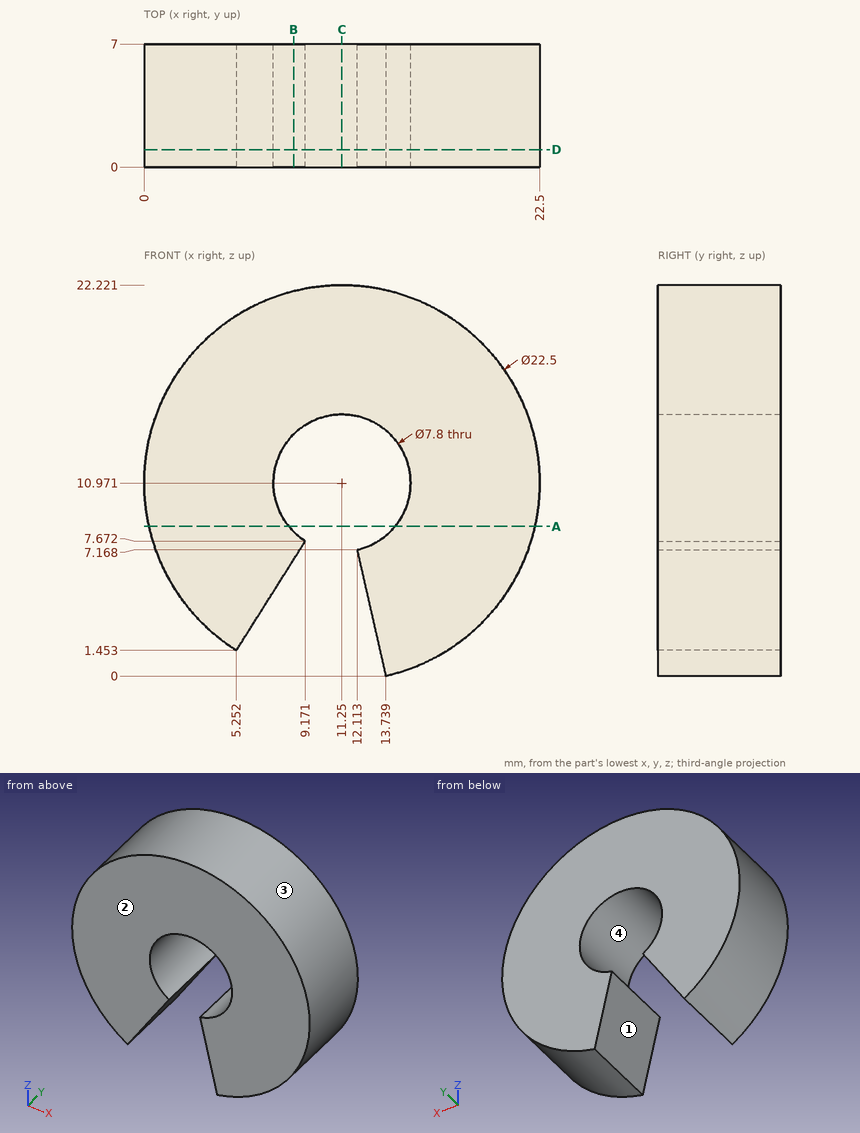
Geometry check sheet. Reference: drawing and pictorial views, mm from the part's lowest x, y, z. Coordinates: 2 decimals unless noted, no trailing zeros. Order: outer loops, then holes, each group sorted by start corner. A loop starts at its lowest first (then second) coordinate and runs counter-clockwise, first axis right, second up.
Item 1: Section check A-A (z = 8.5). Enter the section's corners in (x, y) (1 decimal).
Item 2: Mould release check, pull along Z, two halves, no side actions. Record for the marked faces 1, 2, 3 and 4: released by +Z, released by -Z, zero draft, split by the parting line, or undercut.
Item 3: Section check B-B (x = 8.5). Enter the section's corners in (y, z) (1 decimal).
Item 4: Scan lines: line 1 along Z through (x, y) = (11.25, 2.75); line 2 along Z through (x, y) = (8.75, 3.75) (1 decimal); line 3 along X through (y, z) = (3.5, 5) (1 decimal). Record each from-to range of solid material in increasing order.
Item 5: Depth check by flat-ended pin: pin 1 (5 mm diameter, centred on x = 14.5, z = 14, fed in from -Y); pin 2 (4 mm diameter, centred on y = 3.5, z = 4, fed in from -X); pin 3 (4.5 mm diameter, centred on x = 11.25, z = 10.97, fed in from -Y); pin 4 (1 mm diameter, centred on x = 20, y = 3, fed in from +Z). Enter the tip coordinate at first touch or a pass-through.
Item 6: Section check C-C (x = 11.25). Enter the section's corners in (y, z).
Item 7: Section check D-D (y = 1). Enter the section's corners in (x, z), plus the area to 3 significant figures.
Check sheet entries:
1. outline: (0.3, 0) - (8.2, 0) - (8.2, 7) - (0.3, 7) - close; (14.3, 0) - (22.2, 0) - (22.2, 7) - (14.3, 7) - close
2. face 1: released by -Z
2. face 2: zero draft
2. face 3: split by the parting line
2. face 4: undercut
3. outline: (0, 6.6) - (7, 6.6) - (7, 8.2) - (0, 8.2) - close; (0, 13.7) - (7, 13.7) - (7, 21.9) - (0, 21.9) - close
4. line 1: z = 14.87 to 22.22
4. line 2: z = 7 to 8, 14 to 21.9
4. line 3: x = 1.7 to 7.5, 12.6 to 20.8
5. pin 1: stops at y = 0
5. pin 2: stops at x = 1.16
5. pin 3: passes through
5. pin 4: stops at z = 18.62
6. outline: (0, 14.87) - (7, 14.87) - (7, 22.22) - (0, 22.22) - close
7. outline: (5.25, 1.45) - (9.17, 7.67) arc R3.9 cw (long way) to (12.11, 7.17) - (13.74, 0) arc R11.25 ccw (long way) to start
7. area: 306 mm2
